Answer from the drawing. Dimensions are ordinates in mm from the lowest x, y and z of the part. A direction names the side the tool comes from. Coordinates: 2 decimals unless noted, no trailing zeros. Write each loop counter-clockwise with the first axis right and the second up, starting at its lowest first coordinate (ties: lowest second). Pieces come first, ordered by that corner, then holes. Notation, with made-up numbers: M 23.5,-17 L 73.5,-17 A25 cw 73.5,1 Z; hole C -23.75,29.25 d5. An arc over 180 degrees is marked long. Put each result on its own line as item: value. Start each with the question number.
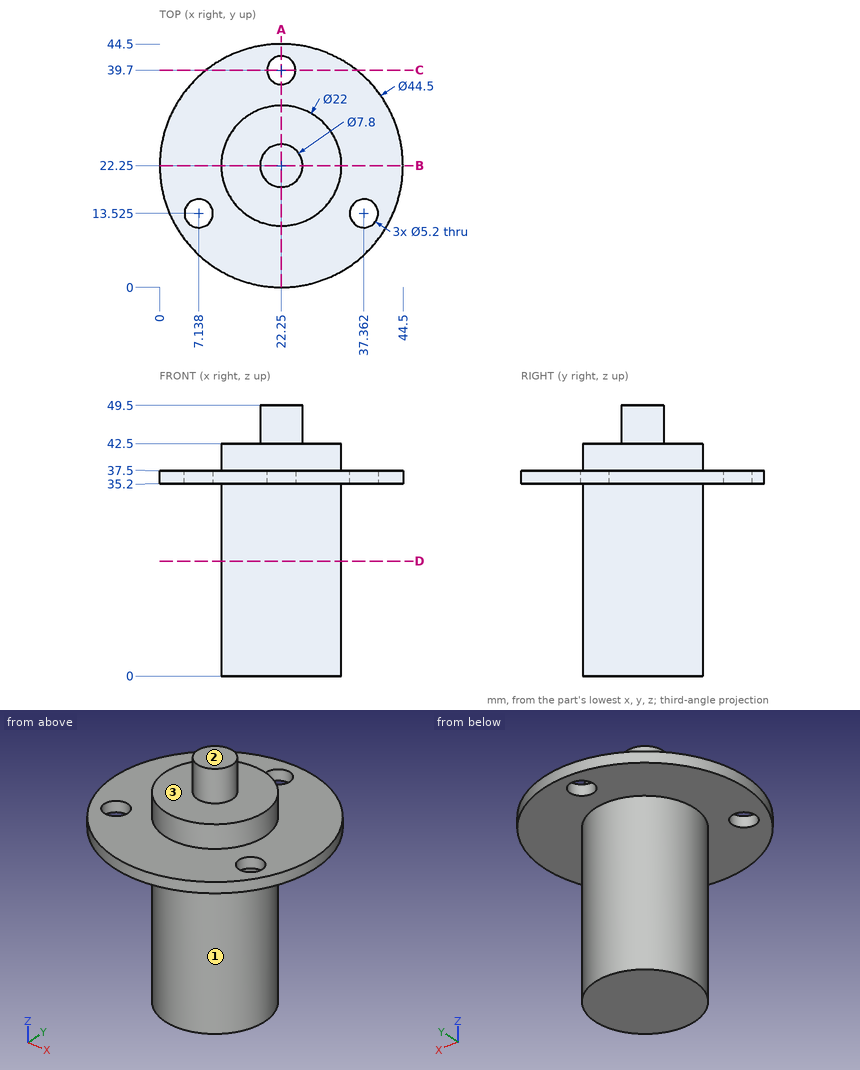
1) A cutting plane is placed at C-C on y = 39.7. Write down the section's boundary in (x, z).
2) Straight lines are drawn through the part: probe 1 along Y at (x, z) = (22.25, 35.8); probe 2 along X at (y, z) = (12.5, 37); probe 3 along Z at (x, y) = (39, 29). For each, find the intervals that lie inside material, in ascending order.
3) A cutting plane is placed at A-A on x = 22.25. Write down the section's boundary in (y, z).
4) For the marked faces 1, 2 and 3, determine the directions among +Z, -Z, +X, -X, +Y, -Y from which every point of the face is accessible in a straight line to the end or side of a thin tool.
5) Given pin 1 Ø22 at (x, y) = (21, 17.5) entering from +Z; pin 2 Ø12 at (x, y) = (38, 14.5) entering from +Z; pin 3 Ø8 at (x, z) = (19, 9.5) entering from -Y; pin 4 Ø5 at (x, z) = (31, 21.5) entering from +Y, each flat-ended and moving along its own axis, determine where each tip first touches the part or whether it passes through.
6) A cutting plane is placed at D-D on z = 21. Write down the section's boundary in (x, y), then the cut area to 3 significant figures.
7) A cutting plane is placed at B-B on y = 22.25. Write down the section's boundary in (x, z).
Answers follow:
1. outline: M 8.45,35.2 L 19.65,35.2 L 19.65,37.5 L 8.45,37.5 Z; M 24.85,35.2 L 36.05,35.2 L 36.05,37.5 L 24.85,37.5 Z
2. probe 1: y = 0 to 37.1, 42.3 to 44.5
2. probe 2: x = 2.25 to 4.75, 9.53 to 34.97, 39.75 to 42.25
2. probe 3: z = 35.2 to 37.5
3. outline: M 0,35.2 L 11.25,35.2 L 11.25,0 L 33.25,0 L 33.25,35.2 L 37.1,35.2 L 37.1,37.5 L 33.25,37.5 L 33.25,42.5 L 26.15,42.5 L 26.15,49.5 L 18.35,49.5 L 18.35,42.5 L 11.25,42.5 L 11.25,37.5 L 0,37.5 Z; M 42.3,35.2 L 44.5,35.2 L 44.5,37.5 L 42.3,37.5 Z
4. face 1: -Z
4. face 2: +Z, +X, -X, +Y, -Y
4. face 3: +Z
5. pin 1: stops at z = 49.5
5. pin 2: stops at z = 37.5
5. pin 3: stops at y = 11.25
5. pin 4: stops at y = 31.3
6. outline: C 22.25,22.25 d22
6. area: 380 mm²
7. outline: M 0,35.2 L 11.25,35.2 L 11.25,0 L 33.25,0 L 33.25,35.2 L 44.5,35.2 L 44.5,37.5 L 33.25,37.5 L 33.25,42.5 L 26.15,42.5 L 26.15,49.5 L 18.35,49.5 L 18.35,42.5 L 11.25,42.5 L 11.25,37.5 L 0,37.5 Z
